```python
from build123d import *

# Parameters (mm, degrees)
BASE_DEPTH        = 1.4
BASE_DEPTH_BACK   = 1.4
BOSS_BLOC_G_DEPTH = 1.9
BOSS_START        = 1.9
BOSS_BLOC_D_DEPTH = 1.9


with BuildPart() as part:
    # Esquisse1 → BASE (new, two sides: drawn at the far end of the back side and taken through both)
    with BuildSketch(Plane(origin=(-65.300145961, -64.810459708, 252.692395796), x_dir=(-0.005843789485583505, 0.9998687257320568, 0.015112293915923657), z_dir=(0.9326954207343167, 1.4198852059309815e-15, 0.3606650137471557)).offset(-BASE_DEPTH_BACK)):
        with BuildLine():
            ThreePointArc((-13.905835762, -115.811989231), (-12.476603332, -119.757071622), (-10.803035184, -115.909273542))
            Line((-10.803035184, -115.909273542), (-12.597966981, -78.341921007))
            Line((-12.597966981, -78.341921007), (-13.097966981, -78.341921007))
            Line((-13.097966981, -78.341921007), (-13.097966981, -76.095588858))
            Line((-13.097966981, -76.095588858), (-10.086767597, -76.095588858))
            Line((-10.086767597, -76.095588858), (-10.086767597, -75.095588858))
            Line((-10.086767597, -75.095588858), (-13.905835762, -75.095588858))
            Line((-13.905835762, -75.095588858), (-13.905835762, -115.811989231))
        make_face()
    extrude(amount=BASE_DEPTH + BASE_DEPTH_BACK)

    # Esquisse2 → BOSS BLOC G (add)
    with BuildSketch(Plane(origin=(29.50317012, 0, 11.408613166), x_dir=(0.36066501374715604, 0, -0.9326954207343167), z_dir=(0.9326954207343167, 0, 0.36066501374715604))):
        with BuildLine():
            ThreePointArc((-142.624687975, -74.263433448), (-143.050736773, -75.335140044), (-142.590186903, -76.392479357))
            ThreePointArc((-142.590186903, -76.392479357), (-140.963090095, -76.690850279), (-140.050933684, -75.310835817))
            ThreePointArc((-140.050933684, -75.310835817), (-140.985527386, -73.921477793), (-142.624687975, -74.263433448))
        make_face()
    extrude(amount=BOSS_BLOC_G_DEPTH)

    # Esquisse3 → BOSS BLOC D (add)
    with BuildSketch(Plane(origin=(26.891622942, 0, 10.398751127), x_dir=(-0.36066501374715587, 0, 0.9326954207343167), z_dir=(-0.9326954207343167, 0, -0.36066501374715587)).offset(BOSS_START)):
        with BuildLine():
            ThreePointArc((143.050933684, -75.310835817), (142.940291708, -74.745429519), (142.624687975, -74.263433448))
            ThreePointArc((142.624687975, -74.263433448), (140.051130596, -75.28653159), (142.590186903, -76.392479357))
            ThreePointArc((142.590186903, -76.392479357), (142.930948146, -75.898679407), (143.050933684, -75.310835817))
        make_face()
    extrude(amount=-BOSS_BLOC_D_DEPTH)


solid = part.part
```
The listing builds one solid part. Answer for the finished solid, in the listing's coordinates (mm). Coordinates: 2 decimals unless noted, no trailing zeros. Write each loop counter-clockwise with the first axis right and the second up, starting at its lowest first coordinate (ties: lowest second). Pieces come first, ordered by that corner, then holes. Notation, with made-up numbers: (84, 80.5) -> (142, 80.5) arc R20 ccw to (142, 96.5) -> close; hole circle Ø5 at (80, 8.25). An arc over 180 degrees is marked (long way). Write each question's results on one line, items separated by ' | '. Start each with the question number.
1) A cutting plane is placed at C-C (z = 170). Determine the outline of the cut face in (x, y).
2) Straight lines are drawn through the part: probe 1 along Y at (x, z) = (-35.5, 173.5); probe 2 along Z at (x, y) = (-38, -74.9); probe 3 along Y at (x, z) = (-34.5, 176.5). For each, find the intervals that lie inside material, in ascending order.
3) Flat-ended cylindrical pins translate along their axes: pin 1 Ø6 at (x, z) = (-37, 178) entering from +Y; pin 2 Ø2 at (y, z) = (-75.5, 175.5) entering from +X; pin 3 Ø1.5 at (x, z) = (-31.5, 168.5) entering from -Y. Find the tip coordinate at first contact, or state that the pin passes through.
4) A cutting plane is placed at B-B (z = 148.5). Determine the outline of the cut face in (x, y), then the cut area to 3 significant figures.
5) A cutting plane is placed at A-A (x = -37.25). Determine the outline of the cut face in (y, z).
Values follow:
1) outline: (-34.82, -77.29) -> (-31.82, -77.27) -> (-31.82, -75.45) -> (-34.82, -75.52) -> close
2) probe 1: -77.35 to -75.75 | probe 2: 181.48 to 182.55 | probe 3: -77.39 to -75.9
3) pin 1: y = -75.86 | pin 2: x = -33.58 | pin 3: y = -77.26
4) outline: (-26.51, -76.92) -> (-23.51, -76.9) -> (-23.51, -73.98) -> (-26.51, -74.05) -> close | area: 8.69 mm²
5) outline: (-77.5, 182.79) -> (-77.4, 176.27) -> (-75.95, 176.27) -> (-76.14, 179.34) -> (-76.64, 179.33) -> (-76.67, 181.74) -> (-73.66, 181.79) -> (-73.68, 182.86) -> close
